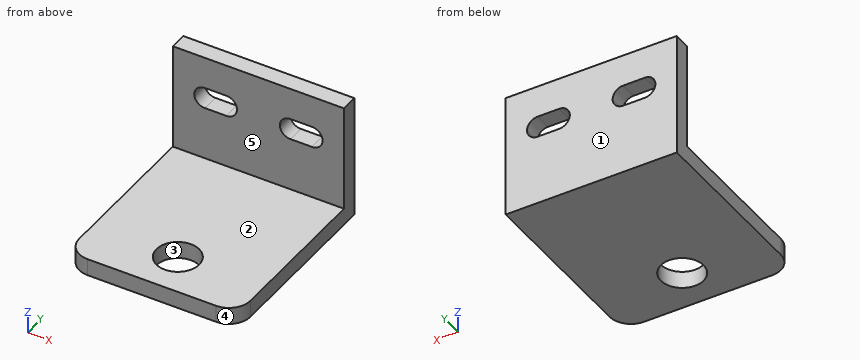
from build123d import *

# Parameters (mm, degrees)
F1_DEPTH = 4
F2_W     = 40
F2_H     = 4
F3_DEPTH = 25
F5_DEPTH = 25
F6_R     = 5
F7_DEPTH = 25


with BuildPart() as f1:
    # F0 (on Top) → F1 (new body)
    with BuildSketch(Plane.XY):
        with BuildLine():
            Line((-35, 0), (-5, 0))
            ThreePointArc((-5, 0), (-1.464466, 1.464466), (0, 5))
            Line((0, 5), (0, 45))
            Line((0, 45), (-40, 45))
            Line((-40, 45), (-40, 5))
            ThreePointArc((-40, 5), (-38.535534, 1.464466), (-35, 0))
        make_face()
    extrude(amount=F1_DEPTH)

    # F2 (on face) → F3 (join)
    with BuildSketch(Plane.XY.offset(4)):
        with Locations((-20, 43)):
            Rectangle(F2_W, F2_H)
    extrude(amount=F3_DEPTH)

    # F4 (on face) → F5 (cut)
    with BuildSketch(Plane(origin=(0, 45, 0), x_dir=(-1, 0, 0), z_dir=(0, 1, 0))):
        with BuildLine():
            ThreePointArc((25, 19), (25.732233, 17.232233), (27.5, 16.5))
            Line((27.5, 16.5), (32.5, 16.5))
            ThreePointArc((32.5, 16.5), (34.267767, 17.232233), (35, 19))
            ThreePointArc((35, 19), (34.267767, 20.767767), (32.5, 21.5))
            Line((32.5, 21.5), (27.5, 21.5))
            ThreePointArc((27.5, 21.5), (25.732233, 20.767767), (25, 19))
        make_face()
        with BuildLine():
            ThreePointArc((5, 19), (5.732233, 17.232233), (7.5, 16.5))
            Line((7.5, 16.5), (12.5, 16.5))
            ThreePointArc((12.5, 16.5), (14.267767, 17.232233), (15, 19))
            ThreePointArc((15, 19), (14.267767, 20.767767), (12.5, 21.5))
            Line((12.5, 21.5), (7.5, 21.5))
            ThreePointArc((7.5, 21.5), (5.732233, 20.767767), (5, 19))
        make_face()
    extrude(amount=-F5_DEPTH, mode=Mode.SUBTRACT)

    # F6 (on face) → F7 (cut)
    with BuildSketch(Plane(origin=(0, 0, 0), x_dir=(1, 0, 0), z_dir=(0, 0, -1))):
        with Locations((-20, -10)):
            Circle(F6_R)
    extrude(amount=-F7_DEPTH, mode=Mode.SUBTRACT)


solid = f1.part
Design review of the part built by this model. Coordinates are the model's own, in mm. Face numbers are marked on the shaded views. A direction names the side the tool comes from. Round coordinates to 2 decimals unless told otherwise and drop trailing zeros. Write each loop counter-clockwise with the first axis right and the second up, starting at its lowest first coordinate (ties: lowest second). Pieces come first, ordered by that corner, then holes. Notation, with made-up numbers: M -10,64 L 19,64 A13 cw 19,71 Z; hole C 14.25,-11 d5. An arc over 180 degrees is marked long. One line per item, written item: value. Start each with the question number.
1. Draft analysis for pull direction X (two halves, no side actions). For the marked faces 3, 4 and 5, state which applies: pulls with the +X half, pulls with the -X half, needs draft (parallel to the pull), parting line crosses it, or undercut.
2. Take a section at A-A on x = -17. State the section outline as (y, z) points, then the cut area to 3 significant figures.
3. For the marked faces 1 and 2, list the 3-axis set-ups (+Z, -Z, +X, -X, +Y, -Y) from which the entire face can be reached by the end or side of a thin tool; tool diameter is ignored.
4. Take a section at C-C on x = -6. State the section outline as (y, z) points.
5. To check wall thickness, follow probe 1 along X at (y, z) = (10, 3.25); probe 2 along Y at (x, z) = (-20, 2.45); probe 3 along Z at (x, y) = (-33, 9). State the ranges of each line that lie inside material, in increasing order. Write a range as from..to.
6. Take a section at B-B on y = 10. State the section outline as (x, z) points.
7. Take a section at D-D on z = 14.5. State the section outline as (x, y) points.
8. Clearance check with flat-ended pins moving along their axes: P1, Ø20, axis at x = -27.5, y = 26, coming from the +Z side; P2, Ø6, axis at x = -33, z = 18, coming from the -Y side; P3, Ø6, axis at y = 21.5, z = 8.5, coming from the +X side. State where each tip first meets the part, or that it passes through.
Computed:
1. face 3: undercut
1. face 4: pulls with the +X half
1. face 5: needs draft
2. outline: M 0,0 L 6,0 L 6,4 L 0,4 Z; M 14,0 L 45,0 L 45,29 L 41,29 L 41,4 L 14,4 Z
2. area: 248 mm²
3. face 1: +Z, -Z, +X, -X, +Y
3. face 2: +Z, +X, -X, -Y
4. outline: M 0,0 L 45,0 L 45,17 L 41,17 L 41,4 L 0,4 Z; M 41,21 L 45,21 L 45,29 L 41,29 Z
5. probe 1: x = -40..-25, -15..0
5. probe 2: y = 0..5, 15..45
5. probe 3: z = 0..4
6. outline: M -40,0 L -25,0 L -25,4 L -40,4 Z; M -15,0 L 0,0 L 0,4 L -15,4 Z
7. outline: M -40,41 L 0,41 L 0,45 L -40,45 Z
8. P1: stops at z = 4
8. P2: stops at y = 41
8. P3: passes through
